from build123d import *

# Parameters (mm, degrees)
SKETCH1_W            = 270
SKETCH1_H            = 27
BASE_FLANGE1_DEPTH   = 1
EDGE_FLANGE1_DEPTH   = 27
EDGE_FLANGE2_DEPTH   = 27
M5_CLEARANCE_HOLE1_D = 5.5


# Sheet-metal steps are written as plain solids
with BuildPart() as part:
    # Sketch1 → Base-Flange1 (new body)
    with BuildSketch(Plane.XY):
        Rectangle(SKETCH1_W, SKETCH1_H)
    extrude(amount=-BASE_FLANGE1_DEPTH)

    # Edge-Flange1 section (across the edge) → Edge-Flange1 (add)
    with BuildSketch(Plane(origin=(136, 13.5, -1), x_dir=(-1, 0, 0), z_dir=(0, -1, 0))):
        with BuildLine():
            Line((-1, 1), (-1, 41))
            Line((-1, 41), (0, 41))
            Line((0, 41), (0, 1))
            ThreePointArc((0, 1), (0.292893219, 0.292893219), (1, 0))
            Line((1, 0), (1, -1))
            ThreePointArc((1, -1), (-0.414213562, -0.414213562), (-1, 1))
        make_face()
    extrude(amount=EDGE_FLANGE1_DEPTH)

    # Edge-Flange2 section (across the edge) → Edge-Flange2 (add)
    with BuildSketch(Plane(origin=(-136, -13.5, -1), x_dir=(1, 0, 0), z_dir=(0, 1, 0))):
        with BuildLine():
            Line((-1, 1), (-1, 26))
            Line((-1, 26), (0, 26))
            Line((0, 26), (0, 1))
            ThreePointArc((0, 1), (0.292893219, 0.292893219), (1, 0))
            Line((1, 0), (1, -1))
            ThreePointArc((1, -1), (-0.414213562, -0.414213562), (-1, 1))
        make_face()
    extrude(amount=EDGE_FLANGE2_DEPTH)

    # M5 Clearance Hole1 (through all)
    with Locations(Plane.XY):
        with Locations((82, 5.5), (-82, 5.5)):
            Hole(M5_CLEARANCE_HOLE1_D / 2)


solid = part.part
The listing builds one solid part. Answer for the finished solid, in the listing's coordinates (mm). A direction names the side the tool comes from. Coordinates: 2 decimals unless noted, no trailing zeros. Write each loop counter-clockwise with the first axis right and the second up, starting at its lowest first coordinate (ties: lowest second). Pieces come first, ordered by that corner, then holes. Notation, with made-up numbers: (70, 49.5) - (87, 49.5) arc R18 cw to (87, 74.5) - close; hole circle Ø11 at (66.25, 47.25). An arc over 180 degrees is marked (long way). Answer as CSV lines item,"result".
1. Find section B-B (y = 5.5). Give the vertices of the cut face in (x, z), plus the area to 3 significant figures.
Computed values:
outline,"(-137, -27) - (-136, -27) - (-136, -2) arc R1 cw to (-135, -1) - (-84.75, -1) - (-84.75, 0) - (-135, 0) arc R2 ccw to (-137, -2) - close; (-79.25, -1) - (79.25, -1) - (79.25, 0) - (-79.25, 0) - close; (84.75, -1) - (135, -1) arc R1 cw to (136, -2) - (136, -42) - (137, -42) - (137, -2) arc R2 ccw to (135, 0) - (84.75, 0) - close"
area,"329 mm²"
2. Given P1, Ø1.1, axis at x = -136.5, y = -2, coming from the -Z side; P2, Ø12, axis at x = 20.5, y = -2, coming from the -Z side, each flat-ended and moving along its own axis, determine where each tip first touches the part or whether it passes through.
Computed values:
P1,"stops at z = -27"
P2,"stops at z = -1"
3. Find section C-C (z = -13). Give the vertices of the cut face in (x, y).
Computed values:
outline,"(-137, -13.5) - (-136, -13.5) - (-136, 13.5) - (-137, 13.5) - close; (136, -13.5) - (137, -13.5) - (137, 13.5) - (136, 13.5) - close"
4. Determine the mould class of faces 1 (the flat face through (-2, 0, 0)), 2 (the cylindrical face through (84.747, 5.621, -0.507)) for opening direction Y: +Y half, -Y half, draft (parallel to the pull), parting line (faces both ways), or undercut.
Computed values:
face 1,"draft"
face 2,"undercut"
5. Straight lines are drawn through the part: line 1 (X direction, y = 7, z = -8.5); line 2 (Y direction, x = -82, z = -0.55); line 3 (Z direction, x = -39, y = -1.25). For each, find the intervals that lie inside material, in ascending order. Write a range as [from, to].
Computed values:
line 1,"x = [-137, -136], [136, 137]"
line 2,"y = [-13.5, 2.75], [8.25, 13.5]"
line 3,"z = [-1, 0]"
6. Find section D-D (y = -8.5). Give the vertices of the cut face in (x, z).
Computed values:
outline,"(-137, -27) - (-136, -27) - (-136, -2) arc R1 cw to (-135, -1) - (135, -1) arc R1 cw to (136, -2) - (136, -42) - (137, -42) - (137, -2) arc R2 ccw to (135, 0) - (-135, 0) arc R2 ccw to (-137, -2) - close"
7. A tool of negligible diameter and unlimited length cuts with its end or side. For faces 3 (the flat face through (137, 0, -22)), 4 (the flat face through (-2, 0, -1)), from which of +Z, -Z, +X, -X, +Y, -Y can it reach the whole face along a straight path? Write none if from no direction.
Computed values:
face 3,"+Z, -Z, +X, +Y, -Y"
face 4,"-Z, +Y, -Y"
8. Find section A-A (x = -82). Give the vertices of the cut face in (y, z).
Computed values:
outline,"(-13.5, -1) - (2.75, -1) - (2.75, 0) - (-13.5, 0) - close; (8.25, -1) - (13.5, -1) - (13.5, 0) - (8.25, 0) - close"
